from build123d import *

# Parameters (mm, degrees)
F0_W     = 2.3
F0_H     = 4
F0_W_2   = 5.4
F0_H_2   = 13
F0_W_3   = 1.7
F0_H_3   = 46.8
F0_W_4   = 4
F0_H_4   = 6
F1_DEPTH = 15
F2_R     = 5.5
F3_DEPTH = 1.8


# Not quite as in the source:
# - a feature names something its author has since deleted; it is built from what else it names


with BuildPart() as f1:
    # F0 (on Top) → F1 (new body)
    with BuildSketch(Plane.XY):
        Polygon((0, -23.2), (0, -13), (-1.7, -13), (-1.7, -17), (-1.7, -23.2), align=None)
        with Locations((-2.85, -15)):
            Rectangle(F0_W, F0_H)
        with Locations((2.7, -6.5)):
            Rectangle(F0_W_2, F0_H_2)
        with Locations((-0.85, -46.6)):
            Rectangle(F0_W_3, F0_H_3)
        Polygon((-11.5, -74), (-11.5, -70), (-11.5, -64), (-15.5, -64), (-15.5, -74), align=None)
        with Locations((1.15, -46.6)):
            Rectangle(F0_W, F0_H_3)
        Polygon((2.3, -70), (0, -70), (-1.7, -70), (-11.5, -70), (-11.5, -74), (2.3, -74), align=None)
        Polygon((0, -13), (0, 0), (-4, -13), (-1.7, -13), align=None)
        Polygon((-4, -17), (-4, -13), (-15.5, -13), (-15.5, -17), (-11.5, -17), align=None)
        with Locations((-13.5, -20)):
            Rectangle(F0_W_4, F0_H_4)
    extrude(amount=F1_DEPTH)

    # F2 (on face) → F3 (cut)
    with BuildSketch(Plane.YZ.offset(5.4)):
        with Locations((-6.5, 7.5)):
            Circle(F2_R)
    extrude(amount=-F3_DEPTH, mode=Mode.SUBTRACT)


solid = f1.part
Work out the finished part from the listing and answer in its coordinate system (mm). A direction names the side the tool comes from. Coordinates: 2 decimals unless noted, no trailing zeros. Write each loop counter-clockwise with the first axis right and the second up, starting at its lowest first coordinate (ties: lowest second). Pieces come first, ordered by that corner, then holes. Notation, with made-up numbers: M 59,-30 L 81,-30 A23 ccw 81,-21 Z; hole C 82,-33.75 d11. An arc over 180 degrees is marked long. Use one line per item in the form item = value. Start each with the question number.
1. A tool of negligible diameter and unlimited length cuts with its end or side. For faces 5 (the face through (-7, -17, 7)), 6 (the face through (3, -13, 7)), 7 (the face through (3.6, -7, 8)), from which of +Z, -Z, +X, -X, +Y, -Y can it reach the whole face along a straight path? Write none if from no direction.
2. The part is cut by section A-A (x = -8.5). Give the vertices of the cut face in (y, z).
3. Straight lines are drawn through the part: probe 1 along Y at (x, z) = (-5.75, 1); probe 2 along Z at (x, y) = (4.5, -6.5); probe 3 along X at (y, z) = (-67.5, 3.5). For each, find the intervals that lie inside material, in ascending order. Write a range as from..to.
4. The part is cut by section D-D (x = -13.5). Give the vertices of the cut face in (y, z).
5. The mould has two halves that part along Y. Classify faces 1 (the face through (3, 0, 7)), 2 (the face through (-14, -23, 7)), 3 (the face through (-7, -74, 7)), 4 (the face through (-15.5, -69, 7)): released by +Y, released by -Y, zero draft, split by the parting line, or undercut.
6. The part is cut by section C-C (y = -6.5). Give the vertices of the cut face in (x, z).
7. The part is cut by section B-B (z = 14). Give the vertices of the cut face in (x, y).
8. Each of these flat-tipped pins is pushed along its axis until it touches: P1, Ø8, axis at x = -11.5, z = 11.5, coming from the +Y side; P2, Ø4.5, axis at y = -34.5, z = 5.5, coming from the -X side; P3, Ø2, axis at x = -4.5, y = -57, coming from the -Z side; P4, Ø0.7, axis at x = 1, z = 8, coming from the +Y side. Where does it stop, or does it pass through?
Evaluation:
q1.face_5 = +Z, -Z
q1.face_6 = +Z, -Z, +X
q1.face_7 = +X
q2.outline = M -74,0 L -70,0 L -70,15 L -74,15 Z; M -17,0 L -13,0 L -13,15 L -17,15 Z
q3.probe_1 = -74..-70, -17..-13
q3.probe_2 = 0..2, 13..15
q3.probe_3 = -15.5..-11.5, -1.7..2.3
q4.outline = M -74,0 L -64,0 L -64,15 L -74,15 Z; M -23,0 L -13,0 L -13,15 L -23,15 Z
q5.face_1 = released by +Y
q5.face_2 = undercut
q5.face_3 = released by -Y
q5.face_4 = zero draft
q6.outline = M -2,0 L 5.4,0 L 5.4,2 L 3.6,2 L 3.6,13 L 5.4,13 L 5.4,15 L -2,15 Z
q7.outline = M -15.5,-74 L 2.3,-74 L 2.3,-23.2 L 0,-23.2 L 0,-13 L 5.4,-13 L 5.4,0 L 0,0 L -4,-13 L -15.5,-13 L -15.5,-23 L -11.5,-23 L -11.5,-17 L -1.7,-17 L -1.7,-70 L -11.5,-70 L -11.5,-64 L -15.5,-64 Z
q8.P1 = -13
q8.P2 = -1.7
q8.P3 = through
q8.P4 = 0
